Autodesk Inventor part; units mm, degrees
ref_plane "YZ Plane" through (0, 0, 0) normal (1, 0, 0) x (0, 1, 0)
ref_plane "XZ Plane" through (0, 0, 0) normal (0, 1, 0) x (-1, 0, 0)
ref_plane "XY Plane" through (0, 0, 0) normal (0, 0, 1) x (1, 0, 0)
sketch "Boceto1" plane through (0, 0, 0) normal (0, 1, 0) x (-1, 0, 0)
  circle A0 centre (0, 0) radius 4
  dimension "d0" = 8
extrude "Extrusión1" add sketch "Boceto1" along normal blind 400
thread "Rosca1"
sketch "Boceto2" plane through (0, 400, 0) normal (0, 1, 0) x (1, 0, 0)
  circle A0 centre (0, 0) radius 4
extrude "Extrusión2" cut sketch "Boceto2" against normal blind 23
sketch "Boceto3" plane through (0, 377, 0) normal (0, 1, 0) x (1, 0, 0)
  circle A0 centre (0, 0) radius 4
extrude "Extrusión3" cut sketch "Boceto3" against normal blind 77
properties part number "tornillo"
For this review, take the finished solid that the model builds, in its own axes (mm). Round coordinates to 2 decimals unless told otherwise and drop trailing zeros. Write each loop counter-clockwise with the first axis right and the second up, starting at its lowest first coordinate (ties: lowest second). Pieces come first, ordered by that corner, then holes. Notation, with made-up numbers: (7, 34.25) -> (15, 34.25) arc R14 cw to (15, 57.25) -> close; hole circle Ø10 at (72, -16.5). An arc over 180 degrees is marked (long way). Use one line per item in the form item = value.
1) To check wall thickness, follow L1, parallel to Z at x = -0.5, y = 270; L2, parallel to X at y = 133, z = 3.5; L3, parallel to X at y = 94, z = 2. State the ranges of each line that lie inside material, in increasing order. Write a range as from..to.
Found:
L1 = -3.97..3.97
L2 = -1.94..1.94
L3 = -3.46..3.46
2) Take a section at A-A, the plane y = 257. Write out the cut boundary in (x, z), and give its area (3 significant figures).
Found:
outline = circle Ø8 at (0, 0)
area = 50.3 mm2
3) Clearance check with a flat-ended pin moving along its axis: pin 1 (1 mm diameter, centred on x = -2, y = 258, fed in from +Z). State where the tip first meets the part, or that it passes through.
Found:
pin_1 = 3.71
4) Take a section at C-C, the plane z = 1.25. Write out the cut boundary in (x, y), and give its area (3 significant figures).
Found:
outline = (-3.8, 0) -> (3.8, 0) -> (3.8, 300) -> (-3.8, 300) -> close
area = 2,280 mm2
5) Take a section at B-B, the plane x = 2.5. Write out the cut boundary in (y, z), and give its area (3 significant figures).
Found:
outline = (0, -3.12) -> (300, -3.12) -> (300, 3.12) -> (0, 3.12) -> close
area = 1,870 mm2
